Model file for the job. Use its own axes, mm. A direction names the side the tool comes from. Coordinates: 2 decimals unless noted, no trailing zeros. Order: outer loops, then holes, each group sorted by start corner. A loop starts at its lowest first (then second) coordinate and runs counter-clockwise, first axis right, second up. Notation, with made-up numbers: (4.25, -27) -> (57.25, -27) arc R13 ccw to (57.25, -10) -> close; hole circle Ø11 at (53.25, 33). An arc over 180 degrees is marked (long way). Return JSON: item names as keys, results as strings. Group by question number.
1) Cut at C-C (x = 1.95). Write the cut outline in (y, z), and give its area (3 significant figures).
2) Probe line 1 (Y direction, x = 2.4, z = 0.65); line 2 (X direction, y = 8.25, z = 1.4); line 3 (Y direction, x = 4.15, z = 0.8). List the from-to ranges inside material, lowest first.
3) Which spindle directions (+Z, -Z, +X, -X, +Y, -Y) get a long thin tool onto all of the face, cutting with end or side? Do faces 5 (the flat face through (2, 8.684, 1)), 6 (the flat face through (2, 10, 1.588)). Say none if no direction does.
4) Cut at D-D (x = 4.45). Write the cut outline in (y, z), and give its area (3 significant figures).
5) Cut at B-B (y = 8.5). Write the cut outline in (x, z).
6) Pull direction Y, two halves, no side cores. Call faces 1 (the cylindrical face through (0.65, 0.69, 0.8)), 2 (the flat face through (1.651, 14, 1)), 3 (the flat face through (0, 10, 1)), 4 (the flat face through (2, 3.928, 1)): +Y half, -Y half, draft (parallel to the pull), parting line (faces both ways), or undercut.
7) Cut at A-A (z = 1). Write the cut outline in (x, y), and give its area (3 significant figures).
from build123d import *

# Parameters (mm, degrees)
SKETCH1_W           = 4.8895
SKETCH1_H           = 20.545176785
BOSS_EXTRUDE1_DEPTH = 1.5875
CUT_EXTRUDE1_DEPTH  = 22.178565948
FILLET1_R           = 2.286


with BuildPart() as part:
    # Sketch1 → Boss-Extrude1 (new body)
    with BuildSketch(Plane.XY):
        with Locations((2.44475, 10.272588393)):
            Rectangle(SKETCH1_W, SKETCH1_H)
    extrude(amount=BOSS_EXTRUDE1_DEPTH)

    # Sketch2 → Cut-Extrude1 (cut, through all)
    with BuildSketch(Plane(origin=(0, 0, 0), x_dir=(-1, 0, 0), z_dir=(0, 0, -1))):
        Polygon((-3.2385, 14.195176785), (-3.2385, 12.036176785), (-1.651, 12.036176785), (-1.651, 14.195176785), (-1.651, 15.351361919), (-1.651, 15.678636285), (-1.651, 16.735176785), (-3.2385, 16.735176785), (-3.2385, 15.678636285), (-3.2385, 15.351361919), align=None)
        Polygon((-1.651, 5.223280418), (-1.651, 6.407477123), (-1.651, 8.684242536), (-3.2385, 8.684242536), (-3.2385, 6.407477123), (-3.2385, 5.223280418), (-3.2385, 4.866564699), (-3.2385, 3.927789612), (-1.651, 3.927789612), (-1.651, 4.866564699), align=None)
    extrude(amount=-CUT_EXTRUDE1_DEPTH, mode=Mode.SUBTRACT)

    # Fillet1
    fillet1_edges = [part.edges().sort_by_distance(p)[0] for p in [
        (0, 20.545176785, 0.79375),
        (4.8895, 20.545176785, 0.79375),
        (4.8895, 0, 0.79375),
        (0, 0, 0.79375),
    ]]
    fillet(fillet1_edges, radius=FILLET1_R)


solid = part.part
Answers below:
{
 "1": {"outline": "(0.02, 0) -> (3.93, 0) -> (3.93, 1.59) -> (0.02, 1.59) -> close; (8.68, 0) -> (12.04, 0) -> (12.04, 1.59) -> (8.68, 1.59) -> close; (16.74, 0) -> (20.52, 0) -> (20.52, 1.59) -> (16.74, 1.59) -> close", "area": "17.5 mm^2"},
 "2": {"line 1": "y = 0 to 3.93, 8.68 to 12.04, 16.74 to 20.55", "line 2": "x = 0 to 1.65, 3.24 to 4.89", "line 3": "y = 0.6 to 19.94"},
 "3": {"face 5": "+Z, -Z", "face 6": "+Z, +X, -X, +Y, -Y"},
 "4": {"outline": "(0.94, 0) -> (19.61, 0) -> (19.61, 1.59) -> (0.94, 1.59) -> close", "area": "29.6 mm^2"},
 "5": {"outline": "(0, 0) -> (1.65, 0) -> (1.65, 1.59) -> (0, 1.59) -> close; (3.24, 0) -> (4.89, 0) -> (4.89, 1.59) -> (3.24, 1.59) -> close"},
 "6": {"face 1": "-Y half", "face 2": "undercut", "face 3": "draft", "face 4": "undercut"},
 "7": {"outline": "(0, 2.29) arc R2.29 ccw to (2.29, 0) -> (2.6, 0) arc R2.29 ccw to (4.89, 2.29) -> (4.89, 18.26) arc R2.29 ccw to (2.6, 20.55) -> (2.29, 20.55) arc R2.29 ccw to (0, 18.26) -> close; hole (1.65, 3.93) -> (3.24, 3.93) -> (3.24, 8.68) -> (1.65, 8.68) -> close; hole (1.65, 12.04) -> (3.24, 12.04) -> (3.24, 16.74) -> (1.65, 16.74) -> close", "area": "81.0 mm^2"}
}
